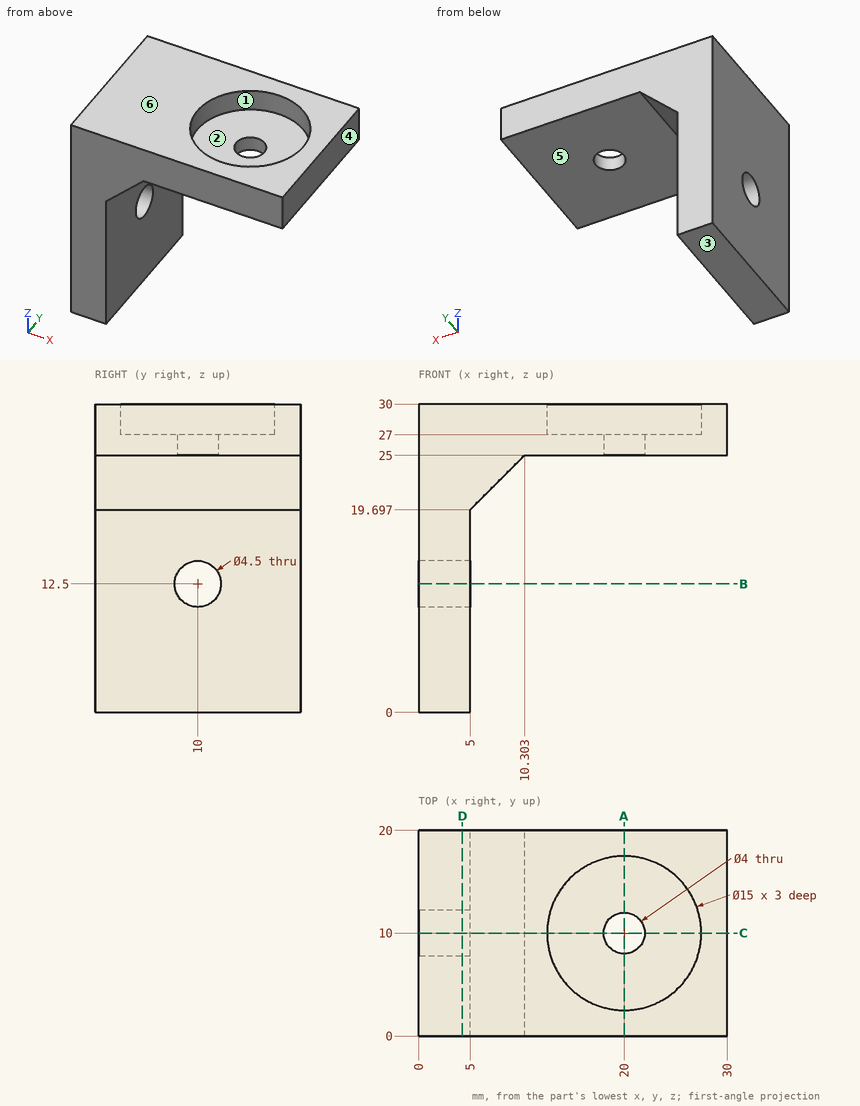
Can you work these out from the drawing? Everything is in mm from the part's minimum corner. A direction names the side the tool comes from. Coordinates: 2 decimals unless noted, no trailing zeros. Order: outer loops, then holes, each group sorted by start corner. A loop starts at its lowest first (then second) coordinate and runs counter-clockwise, first axis right, second up. Notation, with made-up numbers: (57, 77.5) -> (97, 77.5) arc R13 ccw to (97, 86.5) -> close; hole circle Ø3 at (-1.5, -6.5). An arc over 180 degrees is marked (long way). Return JSON: item names as keys, results as strings.
1) If we section it at A-A on x = 20: List the corners of the cut face in (y, z) for me.
Conclusion:
{"outline": "(0, 25) -> (8, 25) -> (8, 27) -> (2.5, 27) -> (2.5, 30) -> (0, 30) -> close; (12, 25) -> (20, 25) -> (20, 30) -> (17.5, 30) -> (17.5, 27) -> (12, 27) -> close"}
2) If we section it at D-D on x = 4.25: List the corners of the cut face in (y, z) for me.
Conclusion:
{"outline": "(0, 0) -> (20, 0) -> (20, 30) -> (0, 30) -> close; hole circle Ø4.5 at (10, 12.5)"}
3) I'm going to push flat-ended pins straight in: P1, Ø4, axis at y = 14.5, z = 18.5, coming from the +X side; P2, Ø10, axis at y = 6, z = 9, coming from the +X side; P3, Ø12, axis at x = 20, y = 10, coming from the -Z side. Where does each tip first touch, or does it pass through?
Conclusion:
{"P1": "stops at x = 5.8", "P2": "stops at x = 5", "P3": "stops at z = 25"}
4) If we section it at C-C on y = 10: List the corners of the cut face in (x, z) for me.
Conclusion:
{"outline": "(0, 0) -> (5, 0) -> (5, 10.25) -> (0, 10.25) -> close; (0, 14.75) -> (5, 14.75) -> (5, 19.7) -> (10.3, 25) -> (18, 25) -> (18, 27) -> (12.5, 27) -> (12.5, 30) -> (0, 30) -> close; (22, 25) -> (30, 25) -> (30, 30) -> (27.5, 30) -> (27.5, 27) -> (22, 27) -> close"}
5) If I drill on probe 1 along Z at (x, y) = (21.75, 12.5); probe 2 along Z at (x, y) = (14.75, 15.5); probe 3 along X at (y, z) = (2.25, 10.25), over which ranges is the centre line in solid material (lowest first)?
Conclusion:
{"probe 1": "z = 25 to 27", "probe 2": "z = 25 to 30", "probe 3": "x = 0 to 5"}
6) Thinking about a two-plate mould opening in X: for the marked faces 1, 2, 3 and 4, which applies, +X half, -X half, draft (parallel to the pull), parting line (faces both ways), or undercut?
Conclusion:
{"face 1": "undercut", "face 2": "undercut", "face 3": "draft", "face 4": "+X half"}
7) If we section it at B-B on z = 12.5: List the corners of the cut face in (x, y) for me, plus the area to 3 significant figures.
Conclusion:
{"outline": "(0, 0) -> (5, 0) -> (5, 7.75) -> (0, 7.75) -> close; (0, 12.25) -> (5, 12.25) -> (5, 20) -> (0, 20) -> close", "area": "77.5 mm²"}
8) On a 3-axis mill with a long thin cutter (end or side, diameter ignored), from which of +Z, -Z, +X, -X, +Y, -Y can I reach the whole of each face in a straight line? I mean the marked faces 5 and 6. Say none if no direction works.
Conclusion:
{"face 5": "-Z, +X, +Y, -Y", "face 6": "+Z, +X, -X, +Y, -Y"}
